```python
from build123d import *

# Parameters (mm, degrees)
ESQUISSE1_R             = 20
BOSS_EXTRU_1_DEPTH      = 20
ESQUISSE2_R             = 2.5
ENL_V_MAT_EXTRU_1_DEPTH = 15
CONG_1_R                = 10
CONG_2_R                = 5
BOSS_EXTRU_2_START      = -5
ESQUISSE3_R             = 20
ESQUISSE3_R_2           = 11.732748591
BOSS_EXTRU_2_DEPTH      = 5


with BuildPart() as part:
    # Esquisse1 → Boss.-Extru.1 (new body)
    with BuildSketch(Plane.XY):
        with BuildLine():
            Line((42, 0), (-42, 0))
            Line((-42, 0), (-42, 5))
            Line((-42, 5), (-22, 5))
            Line((-22, 5), (-22, 30))
            ThreePointArc((-22, 30), (0, 52), (22, 30))
            Line((22, 30), (22, 5))
            Line((22, 5), (42, 5))
            Line((42, 5), (42, 0))
        make_face()
        with Locations((0, 30)):
            Circle(ESQUISSE1_R, mode=Mode.SUBTRACT)
    extrude(amount=BOSS_EXTRU_1_DEPTH)

    # Esquisse2 → Enlèv. mat.-Extru.1 (cut)
    with BuildSketch(Plane(origin=(0, 5, 0), x_dir=(1, 0, 0), z_dir=(0, 1, 0))):
        with Locations(Location((-32, -10, 0), (0, 0, 180))):
            Circle(ESQUISSE2_R)
        with Locations(Location((32, -10, 0), (0, 0, 180))):
            Circle(ESQUISSE2_R)
    extrude(amount=-ENL_V_MAT_EXTRU_1_DEPTH, mode=Mode.SUBTRACT)

    # Congé1
    # the kernel refuses this fillet: 10 mm, written as the material it adds along each edge
    with BuildSketch(Plane(origin=(-22, 5, 0), x_dir=(-1, 0, 0), z_dir=(0, 0, 1))) as cong_1_piece_1_section:
        with BuildLine():
            CenterArc((CONG_1_R, -CONG_1_R), CONG_1_R, 90, 90)
            Line((0, -CONG_1_R), (0, 0))
            Line((0, 0), (CONG_1_R, 0))
        make_face()
    cong_1_piece_1 = extrude(amount=20, mode=Mode.PRIVATE)
    cong_1_piece_1 = cong_1_piece_1 - Plane(origin=(-32, 7.276430514, 10), x_dir=(-1, 0, 0), z_dir=(0, 1, 0)) * Cylinder(2.5, 81, mode=Mode.PRIVATE)
    add(cong_1_piece_1)
    with BuildSketch(Plane(origin=(22, 5, 0), x_dir=(1, 0, 0), z_dir=(0, 0, 1))) as cong_1_piece_2_section:
        with BuildLine():
            CenterArc((CONG_1_R, CONG_1_R), CONG_1_R, 180, 90)
            Line((0, CONG_1_R), (0, 0))
            Line((0, 0), (CONG_1_R, 0))
        make_face()
    cong_1_piece_2 = extrude(amount=20, mode=Mode.PRIVATE)
    cong_1_piece_2 = cong_1_piece_2 - Plane(origin=(32, 7.276430465, 10), x_dir=(-1, 0, 0), z_dir=(0, 1, 0)) * Cylinder(2.5, 80, mode=Mode.PRIVATE)
    add(cong_1_piece_2)

    # Congé2
    cong_2_edges = [part.edges().sort_by_distance(p)[0] for p in [
        (-42, 2.5, 20),
        (42, 2.5, 20),
        (42, 2.5, 0),
        (-42, 2.5, 0),
    ]]
    fillet(cong_2_edges, radius=CONG_2_R)

    # Esquisse3 → Boss.-Extru.2 (add)
    with BuildSketch(Plane.XY.offset(20).offset(BOSS_EXTRU_2_START)):
        with Locations((0, 30)):
            Circle(ESQUISSE3_R)
        with Locations((0, 30)):
            Circle(ESQUISSE3_R_2, mode=Mode.SUBTRACT)
    extrude(amount=BOSS_EXTRU_2_DEPTH)


solid = part.part
```
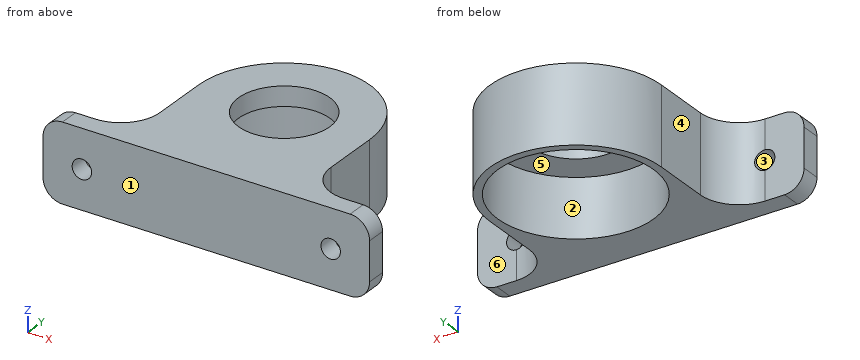
Model file for the job. Use its own axes, mm. Face numbers are marked on the shaded views. A direction names the side the tool comes from. Coordinates: 2 decimals unless noted, no trailing zeros. Loops run counter-clockwise (first coordinate to the right, second up) from the corner with the lowest first, then second, coordinate; pieces in that order, holes last. Notation, with made-up numbers: (-18.5, 12.5) - (18.5, 12.5) arc R22 ccw to (18.5, 40.5) - close; hole circle Ø7 at (10.5, 69). An arc over 180 degrees is marked (long way). Answer as a JSON object with one key per item and string values. Group by question number.
(1) Tool access for the marked faces 4, 5 and 6: list every direction of +Z, -Z, +X, -X, +Y, -Y with a clear straight run to the whole face (end or side of a thin tool).
(2) Cut at D-D (z = 16.25). Give the cut face in (x, y).
(3) Cut at B-B (z = 2.5). Give the cut face in (x, y), then the cut area to 3 significant figures.
(4) Cut at A-A (x = 0). Give the cut face in (y, z).
(5) Flat gauge pins, fed straight in: pin 1 (12 mm diameter, centred on x = -23.5, z = 9.5, fed in from +Y); pin 2 (2 mm diameter, centred on x = 9.5, z = 15, fed in from +Y); pin 3 (1 mm diameter, centred on x = -32.5, z = 13.5, fed in from +Y); pin 4 (3 mm diameter, centred on x = -32, z = 10, fed in from -Y). Where does each tip first touch, or does it go through?
(6) Cut at C-C (y = 35). Give the cut face in (x, z), then the cut area to 3 significant figures.
(7) Probe line 1 along Z through (x, y) = (-32, 3.3); line 2 along Y through (x, z) = (0, 10.25); line 3 along Y through (x, z) = (-6, 5.25). List the from-to ranges inside material, lowest first.
(8) Two-plate mould, pull along Y, no slides. Class the marked faces 1, 2 and 3: released by +Y, released by -Y, zero draft, split by the parting line, or undercut.
Geometry says:
{
 "1": {"face 4": "+Z, -Z, -X, +Y", "face 5": "-Z", "face 6": "+Z, -Z, +X, +Y"},
 "2": {"outline": "(-41.84, 0) - (41.84, 0) - (41.84, 5) - (32, 5) arc R10 cw to (22, 15) - (22, 30) arc R22 ccw to (-22, 30) - (-22, 15) arc R10 cw to (-32, 5) - (-41.84, 5) - close; hole circle Ø23.47 at (0, 30)"},
 "3": {"outline": "(-41.33, 0) - (41.33, 0) - (41.33, 5) - (32, 5) arc R10 cw to (22, 15) - (22, 30) arc R22 ccw to (-22, 30) - (-22, 15) arc R10 cw to (-32, 5) - (-41.33, 5) - close; hole circle Ø40 at (0, 30)", "area": "1,060 mm^2"},
 "4": {"outline": "(0, 0) - (10, 0) - (10, 15) - (18.27, 15) - (18.27, 20) - (0, 20) - close; (41.73, 15) - (50, 15) - (50, 0) - (52, 0) - (52, 20) - (41.73, 20) - close"},
 "5": {"pin 1": "stops at y = 43.33", "pin 2": "stops at y = 50.29", "pin 3": "stops at y = 5", "pin 4": "passes through"},
 "6": {"outline": "(-21.42, 0) - (-19.36, 0) - (-19.36, 15) - (-10.61, 15) - (-10.61, 20) - (-21.42, 20) - close; (10.61, 15) - (19.36, 15) - (19.36, 0) - (21.42, 0) - (21.42, 20) - (10.61, 20) - close", "area": "170 mm^2"},
 "7": {"line 1": "z = 0 to 7.5, 12.5 to 20", "line 2": "y = 0 to 10, 50 to 52", "line 3": "y = 0 to 10.92, 49.08 to 51.17"},
 "8": {"face 1": "released by -Y", "face 2": "undercut", "face 3": "zero draft"}
}
